Source: three-view drawing plus pictorial views. Frame: mm from the lowest corner of the part. A direction names the side the tool comes from. Coordinates: 2 decimals unless noted, no trailing zeros. Loops run counter-clockwise (first coordinate to the right, second up) from the corner with the lowest first, then second, coordinate; pieces in that order, holes last. Notation, with made-up numbers: (71.25, -22) - (118.25, -22) arc R12 ccw to (118.25, -7) - close; hole circle Ø7 at (11.25, 29.25). An arc over 180 degrees is marked (long way). Use CSV: the item, a comma, the result in double quotes. Start each with the question number.
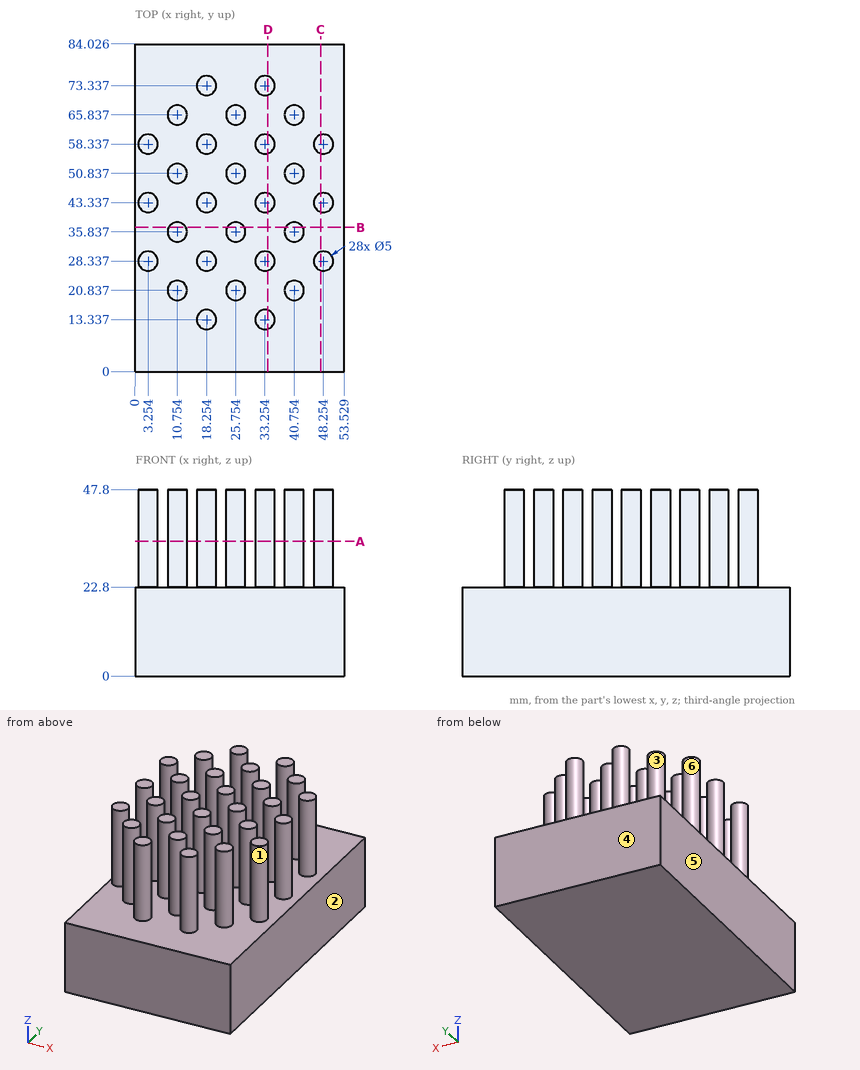
(1) Section B-B on y = 37. Output: boundary loops of the cut face in (x, z), plus the area to 3 significant figures.
(2) Section C-C on x = 47.5. Output: boundary loops of the cut face in (y, z) (1 decimal).
(3) Draft query along Y for the marked faces 3, 4, 5 and 6. Return one class per face: released by +Y, released by -Y, zero draft, split by the parting line, or undercut.
(4) Reachability of the marked faces 1 and 2 from +Z, -Z, +X, -X, +Y, -Y: full face, straight path, thin tool, end or side. Return the list, or none.
(5) Section D-D on x = 34. Output: boundary loops of the cut face in (y, z) (1 decimal), plus the area to 3 significant figures.
(6) Section A-A on z = 34.5. State how many separate pieces and enclosed holes the cut face has.
(7) Ray query, line 1 (Y direction, x = 18, z = 43); line 2 (Y direction, x = 43, z = 32) (1 decimal); line 3 (Z direction, x = 45, y = 68.5). Return the intervals inside material, ascending. Write a range as [from, to].
(8) Pin query (flat end, axial travel): pin 1 Ø5 at (x, z) = (20.5, 31) entering from +Y; pin 2 Ø10 at (y, z) = (10.5, 30) entering from -X; pin 3 Ø8 at (y, z) = (45.5, 40) entering from +X. Return the tip coordinate at first contact, or that it passes through.
Solution:
1,outline,"(0, 0) - (53.53, 0) - (53.53, 22.8) - (42.97, 22.8) - (42.97, 47.8) - (38.54, 47.8) - (38.54, 22.8) - (27.97, 22.8) - (27.97, 47.8) - (23.54, 47.8) - (23.54, 22.8) - (12.97, 22.8) - (12.97, 47.8) - (8.54, 47.8) - (8.54, 22.8) - (0, 22.8) - close"
1,area,"1,550 mm²"
2,outline,"(0, 0) - (84, 0) - (84, 22.8) - (60.7, 22.8) - (60.7, 47.8) - (56, 47.8) - (56, 22.8) - (45.7, 22.8) - (45.7, 47.8) - (41, 47.8) - (41, 22.8) - (30.7, 22.8) - (30.7, 47.8) - (26, 47.8) - (26, 22.8) - (0, 22.8) - close"
3,face 3,"undercut"
3,face 4,"released by +Y"
3,face 5,"zero draft"
3,face 6,"undercut"
4,face 1,"+Z"
4,face 2,"+Z, -Z, +X, +Y, -Y"
5,outline,"(0, 0) - (84, 0) - (84, 22.8) - (75.7, 22.8) - (75.7, 47.8) - (71, 47.8) - (71, 22.8) - (60.7, 22.8) - (60.7, 47.8) - (56, 47.8) - (56, 22.8) - (45.7, 22.8) - (45.7, 47.8) - (41, 47.8) - (41, 22.8) - (30.7, 22.8) - (30.7, 47.8) - (26, 47.8) - (26, 22.8) - (15.7, 22.8) - (15.7, 47.8) - (11, 47.8) - (11, 22.8) - (0, 22.8) - close"
5,area,"2,510 mm²"
6,separate pieces,"28"
6,enclosed holes,"0"
7,line 1,"y = [10.85, 15.82], [25.85, 30.82], [40.85, 45.82], [55.85, 60.82], [70.85, 75.82]"
7,line 2,"y = [19.7, 21.9], [34.7, 36.9], [49.7, 51.9], [64.7, 66.9]"
7,line 3,"z = [0, 22.8]"
8,pin 1,"stops at y = 75.84"
8,pin 2,"stops at x = 15.75"
8,pin 3,"stops at x = 50.75"
